from build123d import *

# Parameters (mm, degrees)
IZIM1_W               = 128
IZIM1_H               = 48
IZIM1_W_2             = 120
IZIM1_H_2             = 40
EKSTR_ZYON_NCE1_DEPTH = 150
KES_EKSTR_ZYON1_REACH = 202.449
IZIM2_R               = 4


with BuildPart() as part:
    # Çizim1 → Ekstrüzyon-İnce1 (new body)
    with BuildSketch(Plane.XY):
        with Locations((-60, 20)):
            Rectangle(IZIM1_W, IZIM1_H)
        with Locations((-60, 20)):
            Rectangle(IZIM1_W_2, IZIM1_H_2, mode=Mode.SUBTRACT)
    extrude(amount=EKSTR_ZYON_NCE1_DEPTH)

    # Çizim2 → Kes-Ekstrüzyon1 (cut, up to next)
    with BuildSketch(Plane(origin=(0, 44, 0), x_dir=(1, 0, 0), z_dir=(0, 1, 0)), mode=Mode.PRIVATE) as kes_ekstr_zyon1_sk1:
        with Locations(Location((-84.5, -75, 0), (0, 0, 180))):
            Circle(IZIM2_R)
    kes_ekstr_zyon1_tool1 = extrude(kes_ekstr_zyon1_sk1.sketch, amount=-KES_EKSTR_ZYON1_REACH, mode=Mode.PRIVATE) & part.part
    # Çizim2 → Kes-Ekstrüzyon1 (cut, up to next)
    with BuildSketch(Plane(origin=(0, 44, 0), x_dir=(1, 0, 0), z_dir=(0, 1, 0)), mode=Mode.PRIVATE) as kes_ekstr_zyon1_sk2:
        with Locations((-35.5, -75)):
            Circle(IZIM2_R)
    kes_ekstr_zyon1_tool2 = extrude(kes_ekstr_zyon1_sk2.sketch, amount=-KES_EKSTR_ZYON1_REACH, mode=Mode.PRIVATE) & part.part
    # Çizim2 → Kes-Ekstrüzyon1 (cut, up to next)
    with BuildSketch(Plane(origin=(0, 44, 0), x_dir=(1, 0, 0), z_dir=(0, 1, 0)), mode=Mode.PRIVATE) as kes_ekstr_zyon1_sk3:
        with Locations(Location((-60, -60, 0), (0, 0, 180))):
            Circle(IZIM2_R)
    kes_ekstr_zyon1_tool3 = extrude(kes_ekstr_zyon1_sk3.sketch, amount=-KES_EKSTR_ZYON1_REACH, mode=Mode.PRIVATE) & part.part
    # Çizim2 → Kes-Ekstrüzyon1 (cut, up to next)
    with BuildSketch(Plane(origin=(0, 44, 0), x_dir=(1, 0, 0), z_dir=(0, 1, 0)), mode=Mode.PRIVATE) as kes_ekstr_zyon1_sk4:
        with Locations((-60, -90)):
            Circle(IZIM2_R)
    kes_ekstr_zyon1_tool4 = extrude(kes_ekstr_zyon1_sk4.sketch, amount=-KES_EKSTR_ZYON1_REACH, mode=Mode.PRIVATE) & part.part
    add(kes_ekstr_zyon1_tool1.solids().sort_by_distance((-84.5, 44, 75))[0], mode=Mode.SUBTRACT)
    add(kes_ekstr_zyon1_tool2.solids().sort_by_distance((-35.5, 44, 75))[0], mode=Mode.SUBTRACT)
    add(kes_ekstr_zyon1_tool3.solids().sort_by_distance((-60, 44, 60))[0], mode=Mode.SUBTRACT)
    add(kes_ekstr_zyon1_tool4.solids().sort_by_distance((-60, 44, 90))[0], mode=Mode.SUBTRACT)


solid = part.part
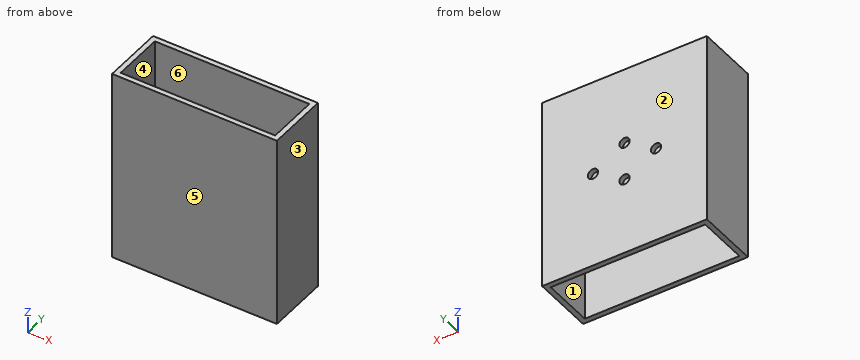
Geometry check sheet. Reference: the model listing, model coordinates, mm. Face numbers are marked on the shaded views. A direction names the side the tool comes from. Round coordinates to 2 decimals unless told otherwise and drop trailing zeros. Write each loop counter-clockwise with the first axis right and the second up, starting at its lowest first coordinate (ties: lowest second). Pieces come first, ordered by that corner, then holes. Notation, with made-up numbers: (42.25, -37.75) -> (53.25, -37.75) arc R21 cw to (53.25, -16.75) -> close; hole circle Ø8 at (71, -14.75). An arc over 180 degrees is marked (long way). One line per item, written item: value. Start each with the question number.
(1) Draft check along Y on the marked faces 3, 4, 5 and 6. Enter one of: +Y half, -Y half, draft (parallel to the pull), parting line (faces both ways), or undercut.
(2) Cross-section at A-A, the plane y = 3. Record the cut outline in (x, z), and give its area (3 significant figures).
(3) Cross-section at B-B, the plane z = 75. Record the cut outline in (x, y).
(4) Cross-section at D-D, the plane x = -112. Record the cut outline in (y, z), and give its area (3 significant figures).
(5) Cross-section at C-C, the plane x = -60. Record the cut outline in (y, z).
(6) Scan lines: line 1 (Z direction, x = -60, y = 42.25); line 2 (X direction, y = 6.5, z = 7); line 3 (Y direction, x = -77, z = 64). Record each from-to range of solid material in increasing order. Write a range as [from, to].
(7) Go/stop test with flat-tipped pins: pin 1 Ø7 at (x, z) = (-84.5, 75) entering from +Y; pin 2 Ø6 at (x, y) = (-19, 5) entering from -Z. Record where each tip stops, or that it passes through.
(8) Access from +Z, -Z, +X, -X, +Y, -Y to the whole of each face (thin tool, end or side, straight path). Record for the marked faces 1 and 2.
Answer:
1. face 3: draft
1. face 4: undercut
1. face 5: -Y half
1. face 6: undercut
2. outline: (-124, 0) -> (-120, 0) -> (-120, 150) -> (-124, 150) -> close; (0, 0) -> (4, 0) -> (4, 150) -> (0, 150) -> close
2. area: 1,200 mm²
3. outline: (-124, -4) -> (4, -4) -> (4, 44) -> (-31.5, 44) -> (-31.5, 40) -> (0, 40) -> (0, 0) -> (-120, 0) -> (-120, 40) -> (-88.5, 40) -> (-88.5, 44) -> (-124, 44) -> close; (-80.5, 40) -> (-39.5, 40) -> (-39.5, 44) -> (-80.5, 44) -> close
4. outline: (-4, 0) -> (0, 0) -> (0, 150) -> (-4, 150) -> close; (40, 0) -> (44, 0) -> (44, 150) -> (40, 150) -> close
4. area: 1,200 mm²
5. outline: (-4, 0) -> (0, 0) -> (0, 150) -> (-4, 150) -> close; (40, 0) -> (44, 0) -> (44, 56) -> (40, 56) -> close; (40, 64) -> (44, 64) -> (44, 86) -> (40, 86) -> close; (40, 94) -> (44, 94) -> (44, 150) -> (40, 150) -> close
6. line 1: [0, 56], [64, 86], [94, 150]
6. line 2: [-124, -120], [0, 4]
6. line 3: [-4, 0], [40, 44]
7. pin 1: y = 0
7. pin 2: through
8. face 1: +Z, -Z
8. face 2: +Z, -Z, +X, -X, +Y
